The listing builds one solid part. Answer for the finished solid, in the listing's coordinates (mm). Face numbers are marked on the shaded views. A direction names the side the tool comes from. Coordinates: 2 decimals unless noted, no trailing zeros. Order: outer loops, then holes, each group sorted by start corner. A loop starts at its lowest first (then second) coordinate and runs counter-clockwise, first axis right, second up. Notation, with made-up numbers: (31, 51) -> (43, 51) arc R23 cw to (43, 85) -> close; hole circle Ø9 at (-18, 13.5). An arc over 180 degrees is marked (long way). Return JSON: item names as keys, results as strings.
```python
from build123d import *

# Parameters (mm, degrees)
SKETCH1_R           = 3
BOSS_EXTRUDE2_DEPTH = 1
FILLET3_R           = 1
SKETCH4_W           = 0.338616022
SKETCH4_H           = 2.447710107
BOSS_EXTRUDE3_DEPTH = 5


with BuildPart() as part:
    # Sketch1 → Boss-Extrude2 (new body)
    with BuildSketch(Plane(origin=(0, 0, 0), x_dir=(1, 0, 0), z_dir=(0, 1, 0))):
        with Locations(Location((0, 0, 0), (0, 0, 270))):
            Circle(SKETCH1_R)
    extrude(amount=BOSS_EXTRUDE2_DEPTH)

    # Fillet3
    fillet3_edges = [part.edges().sort_by_distance(p)[0] for p in [
        (0, 1, -3),
    ]]
    fillet(fillet3_edges, radius=FILLET3_R - 0.0001)  # a hair under: the kernel refuses the full size

    # Sketch4 → Boss-Extrude3 (add)
    with BuildSketch(Plane(origin=(0, 1, 0), x_dir=(1, 0, 0), z_dir=(0, 1, 0))):
        with Locations((1.02068544, -0.004837371)):
            Rectangle(SKETCH4_W, SKETCH4_H)
        with Locations((-1.02068544, -0.004837371)):
            Rectangle(SKETCH4_W, SKETCH4_H)
    extrude(amount=BOSS_EXTRUDE3_DEPTH)


solid = part.part
```
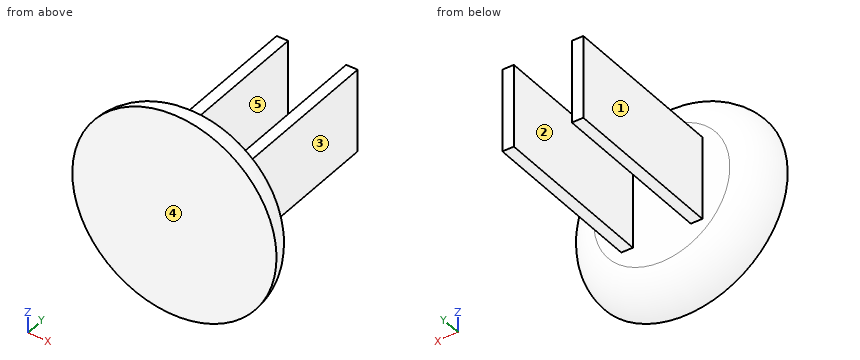
Item 1: Which of the six approach directions +Z, -Z, +X, -X, +Y, -Y give full straight-line access (tool end or side, diameter ignored) to the marked faces 1 and 2?
Answer list:
{"face 1": "+Z, -Z, -X, +Y", "face 2": "+Z, -Z, +Y"}
Item 2: The part is cut by section A-A on y = 4.8. Determine the outline of the cut face in (x, z), plus the area to 3 significant figures.
Answer list:
{"outline": "(-1.19, -1.22) -> (-0.85, -1.22) -> (-0.85, 1.23) -> (-1.19, 1.23) -> close; (0.85, -1.22) -> (1.19, -1.22) -> (1.19, 1.23) -> (0.85, 1.23) -> close", "area": "1.66 mm2"}
Item 3: Determine the mould class of the marked faces 3, 4 and 5 for opening direction X: pulls with the +X half, pulls with the -X half, needs draft (parallel to the pull), parting line crosses it, or undercut.
Answer list:
{"face 3": "pulls with the +X half", "face 4": "needs draft", "face 5": "undercut"}
Item 4: Find the intervals of material crossed by probe 1 along X at (y, z) = (4.7, -0.95); probe 2 along Y at (x, z) = (0, 1); probe 3 along Z at (x, y) = (1, 2.85), in increasing order.
Answer list:
{"probe 1": "-1.19 to -0.85, 0.85 to 1.19", "probe 2": "0 to 1", "probe 3": "-1.22 to 1.23"}
Item 5: Flat-ended cylindrical pins translate along their axes: pin 1 (0.7 mm diameter, centred on y = 4.5, z = 0.5, fed in from +X); pin 2 (2 mm diameter, centred on x = -1, y = 3, fed in from +Z); pin 3 (1 mm diameter, centred on x = 1, y = 2, fed in from -Z). Find the tip coordinate at first contact, or state that the pin passes through.
Answer list:
{"pin 1": "x = 1.19", "pin 2": "z = 1.23", "pin 3": "z = -1.22"}
